from build123d import *

# Parameters (mm, degrees)
BOSS_EXTRUDE1_DEPTH              = 3.175
F_10_0_1935_DIAMETER_HOLE1_D     = 4.9149
F_10_0_1935_DIAMETER_HOLE1_DEPTH = 25.4
F_10_0_1935_DIAMETER_HOLE1_TIP   = 1.476584928


with BuildPart() as part:
    # Sketch1 → Boss-Extrude1 (new body)
    with BuildSketch(Plane(origin=(0, 0, 0), x_dir=(1, 0, 0), z_dir=(0, 1, 0))):
        Polygon((0, 0), (0, 76.2), (25.4, 76.2), (76.2, 25.4), (76.2, 0), align=None)
    extrude(amount=BOSS_EXTRUDE1_DEPTH)

    # #10 (0.1935) Diameter Hole1
    with Locations(Plane(origin=(0, 0, 0), x_dir=(-1, 0, 0), z_dir=(0, -1, 0))):
        with Locations((-12.7, 12.7), (-12.7, 38.1), (-12.7, 63.5), (-38.1, 12.7), (-63.5, 12.7)):
            Hole(F_10_0_1935_DIAMETER_HOLE1_D / 2, depth=F_10_0_1935_DIAMETER_HOLE1_DEPTH)
            with Locations((0, 0, -(F_10_0_1935_DIAMETER_HOLE1_DEPTH + F_10_0_1935_DIAMETER_HOLE1_TIP / 2))):  # 118° drill point
                Cone(0, F_10_0_1935_DIAMETER_HOLE1_D / 2, F_10_0_1935_DIAMETER_HOLE1_TIP, mode=Mode.SUBTRACT)


solid = part.part
Read the model definition and answer for the solid it produces. Units are mm, in the model's axes. Round coordinates to 2 decimals unless told otherwise and drop trailing zeros. Write each loop counter-clockwise with the first axis right and the second up, starting at its lowest first coordinate (ties: lowest second). Pieces come first, ordered by that corner, then holes.
1. The part is cut by section D-D, the plane y = 2.3. Determine the outline of the cut face in (x, z).
2. Determine the mould class of faces 1 (the face through (15.044, 1.61, -13.438)), 2 (the face through (13, 2, -76.2)), 3 (the face through (0, 2, -38)) for opening direction X: pulls with the +X half, pulls with the -X half, needs draft (parallel to the pull), parting line crosses it, or undercut.
3. The part is cut by section C-C, the plane z = -37. Determine the outline of the cut face in (x, y) (3 decimals), then the cut area to 3 significant figures.
4. The part is cut by section B-B, the plane x = 12.7. Determine the outline of the cut face in (y, z) (3 decimals).
5. Straight lines are drawn through the part: L1, parallel to Z at x = 12.7, y = 0.9; L2, parallel to X at y = 1.05, z = -12.7; L3, parallel to X at y = 1.5, z = -11. For each, find the intervals that lie inside material, in ascending order.
6. The part is cut by section A-A, the plane x = 38.1. Determine the outline of the cut face in (y, z) (3 decimals).
Values:
1. outline: (0, -76.2) - (25.4, -76.2) - (76.2, -25.4) - (76.2, 0) - (0, 0) - close; hole circle Ø4.91 at (12.7, -63.5); hole circle Ø4.91 at (12.7, -38.1); hole circle Ø4.91 at (12.7, -12.7); hole circle Ø4.91 at (38.1, -12.7); hole circle Ø4.91 at (63.5, -12.7)
2. face 1: undercut
2. face 2: needs draft
2. face 3: pulls with the -X half
3. outline: (0, 0) - (10.502, 0) - (10.502, 3.175) - (0, 3.175) - close; (14.898, 0) - (64.6, 0) - (64.6, 3.175) - (14.898, 3.175) - close
3. area: 191 mm2
4. outline: (0, -76.2) - (3.175, -76.2) - (3.175, -65.957) - (0, -65.957) - close; (0, -61.043) - (3.175, -61.043) - (3.175, -40.557) - (0, -40.557) - close; (0, -35.643) - (3.175, -35.643) - (3.175, -15.157) - (0, -15.157) - close; (0, -10.243) - (3.175, -10.243) - (3.175, 0) - (0, 0) - close
5. L1: z = -76.2 to -65.96, -61.04 to -40.56, -35.64 to -15.16, -10.24 to 0
5. L2: x = 0 to 10.24, 15.16 to 35.64, 40.56 to 61.04, 65.96 to 76.2
5. L3: x = 0 to 10.93, 14.47 to 36.33, 39.87 to 61.73, 65.27 to 76.2
6. outline: (0, -63.5) - (3.175, -63.5) - (3.175, -15.157) - (0, -15.157) - close; (0, -10.243) - (3.175, -10.243) - (3.175, 0) - (0, 0) - close
